Job drawing, mm, ordinate dimensions from the low corner. One solid piece. A direction names the side the tool comes from. Round coordinates to 2 decimals unless told otherwise and drop trailing zeros. Loops run counter-clockwise (first coordinate to the right, second up) from the corner with the lowest first, then second, coordinate; pieces in that order, holes last.
1) Mould opens along X. For the marked faces 3, 4 and 5 say: +X half, -X half, draft (parallel to the pull), parting line (faces both ways), or undercut.
2) Band-saw the part on C-C, the plane x = 5. Write the cut outline in (y, z).
3) Probe line 1 (X direction, y = 5, z = 4); line 2 (X direction, y = 0.75, z = 7.5); line 3 (Y direction, x = 11, z = 9.5). List the from-to ranges inside material, lowest first.
4) Band-saw the part on D-D, the plane y = 9.75. Write the cut outline in (x, z), then the cut area to 3 significant figures.
5) Band-saw the part on A-A, the plane y = 3.5. Write the cut outline in (x, z), then the cut area to 3 significant figures.
6) Band-saw the part on B-B, the plane z = 7.25. Write the cut outline in (x, y).
7) 3-axis set-ups, long thin cutter, end or side, ignore diameter. For the marked faces 1 and 2: which of +Z, -Z, +X, -X, +Y, -Y reach the whole face in a straight line?
8) Drop a flat-ended pin along its axis: P1, Ø1.1, axis at x = 10.5, y = 0.5, coming from the -Z side. Give the stop position or say it passes through.
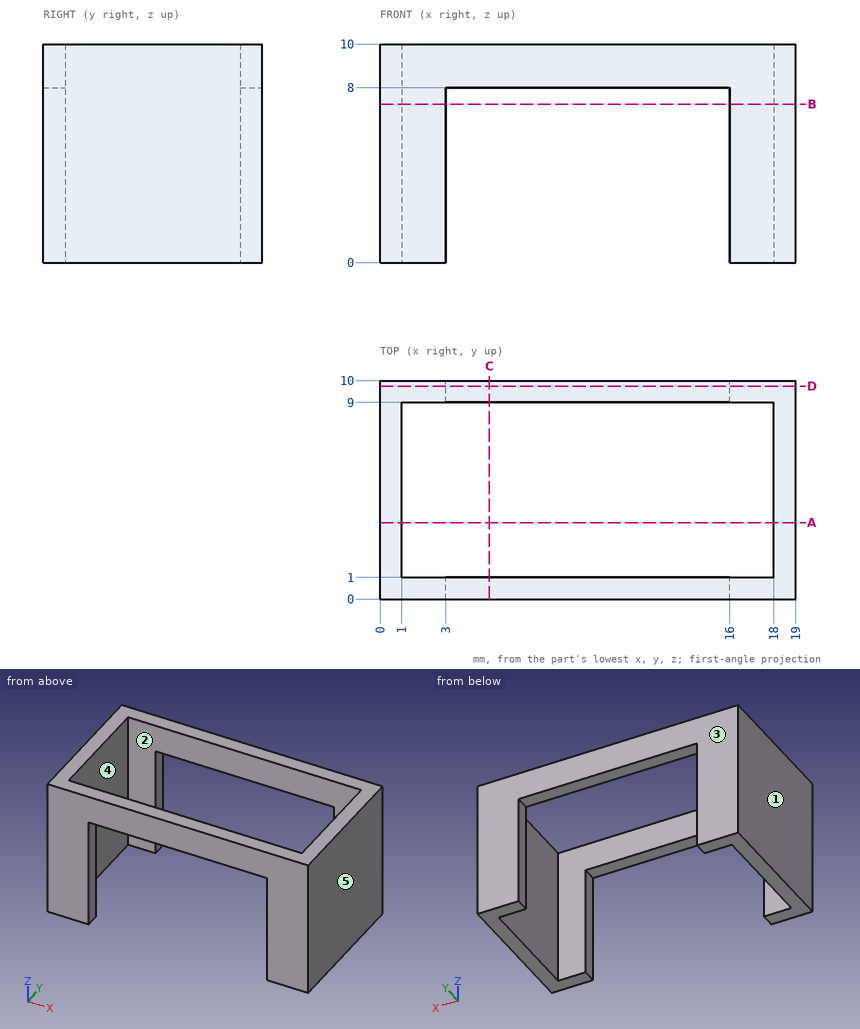
Reported:
1. face 3: draft
1. face 4: undercut
1. face 5: +X half
2. outline: (0, 8) - (1, 8) - (1, 10) - (0, 10) - close; (9, 8) - (10, 8) - (10, 10) - (9, 10) - close
3. line 1: x = 0 to 1, 18 to 19
3. line 2: x = 0 to 3, 16 to 19
3. line 3: y = 0 to 1, 9 to 10
4. outline: (0, 0) - (3, 0) - (3, 8) - (16, 8) - (16, 0) - (19, 0) - (19, 10) - (0, 10) - close
4. area: 86.0 mm2
5. outline: (0, 0) - (1, 0) - (1, 10) - (0, 10) - close; (18, 0) - (19, 0) - (19, 10) - (18, 10) - close
5. area: 20.0 mm2
6. outline: (0, 0) - (3, 0) - (3, 1) - (1, 1) - (1, 9) - (3, 9) - (3, 10) - (0, 10) - close; (16, 0) - (19, 0) - (19, 10) - (16, 10) - (16, 9) - (18, 9) - (18, 1) - (16, 1) - close
7. face 1: +Z, -Z, -X, +Y, -Y
7. face 2: +Z, -Z
8. P1: stops at z = 8
